Read the model definition and answer for the solid it produces. Units are mm, in the model's axes. A direction names the side the tool comes from. Coordinates: 2 decimals unless noted, no trailing zeros. Loops run counter-clockwise (first coordinate to the right, second up) from the corner with the lowest first, then second, coordinate; pieces in that order, holes last. Notation, with made-up numbers: M 41.5,4 L 96.5,4 A8 cw 96.5,14 Z; hole C -40,17.25 d4. An arc over 180 degrees is marked long. Put each result on its own line as item: value.
from build123d import *

# Parameters (mm, degrees)
SKETCH1_R               = 12.7
BOSS_EXTRUDE1_DEPTH     = 44.45
SKETCH5_R               = 12.7
SKETCH5_R_2             = 6.35
BOSS_EXTRUDE2_DEPTH     = 6.35
SKETCH8_W               = 6.35
SKETCH8_H               = 6.35
CUT_EXTRUDE1_DEPTH      = 51.8
CUT_EXTRUDE1_DEPTH_BACK = 51.8


with BuildPart() as part:
    # Sketch1 → Boss-Extrude1 (new body, symmetric)
    with BuildSketch(Plane.XY):
        with BuildLine():
            Line((-59.699595301, -246.884504011), (-38.184359795, -0.964236874))
            ThreePointArc((-38.184359795, -0.964236874), (-38.124009824, -0.108037848), (-38.092623076, 0.749711395))
            ThreePointArc((-38.092623076, 0.749711395), (0, 38.1), (38.092623076, 0.749711395))
            ThreePointArc((38.092623076, 0.749711395), (38.124009824, -0.108037848), (38.184359795, -0.964236874))
            Line((38.184359795, -0.964236874), (59.699595301, -246.884504011))
            ThreePointArc((59.699595301, -246.884504011), (0, -254), (-59.699595301, -246.884504011))
        make_face()
        Circle(SKETCH1_R, mode=Mode.SUBTRACT)
    extrude(amount=BOSS_EXTRUDE1_DEPTH, both=True)

    # Sketch5 → Boss-Extrude2 (add)
    with BuildSketch(Plane.XY.offset(44.45)):
        with BuildLine():
            Line((-223.779910529, -44.577802506), (-54.04268144, -3.827499177))
            ThreePointArc((-54.04268144, -3.827499177), (-42.924981025, 2.041131203), (-35.983316209, 12.522418081))
            ThreePointArc((-35.983316209, 12.522418081), (0, 38.1), (35.983316209, 12.522418081))
            ThreePointArc((35.983316209, 12.522418081), (42.924981025, 2.041131203), (54.04268144, -3.827499177))
            Line((54.04268144, -3.827499177), (223.779910529, -44.577802506))
            ThreePointArc((223.779910529, -44.577802506), (239.972758508, -56.795566669), (242.055998097, -76.973331649))
            ThreePointArc((242.055998097, -76.973331649), (0, -254), (-242.055998097, -76.973331649))
            ThreePointArc((-242.055998097, -76.973331649), (-239.972758508, -56.795566669), (-223.779910529, -44.577802506))
        make_face()
        Circle(SKETCH5_R, mode=Mode.SUBTRACT)
        with Locations((-117.332700629, -48.60079591)):
            Circle(SKETCH5_R_2, mode=Mode.SUBTRACT)
        with Locations((117.332700629, -48.60079591)):
            Circle(SKETCH5_R_2, mode=Mode.SUBTRACT)
    boss_extrude2 = extrude(amount=BOSS_EXTRUDE2_DEPTH)

    # Mirror1: Boss-Extrude2 across plane
    add(boss_extrude2.mirror(Plane.XY))

    # Sketch8 → Cut-Extrude1 (cut, two sides)
    with BuildSketch(Plane.XY) as cut_extrude1_sk:
        with Locations((0, 12.7)):
            Rectangle(SKETCH8_W, SKETCH8_H)
    extrude(amount=CUT_EXTRUDE1_DEPTH, mode=Mode.SUBTRACT)
    extrude(cut_extrude1_sk.sketch, amount=-CUT_EXTRUDE1_DEPTH_BACK, mode=Mode.SUBTRACT)


solid = part.part
1) Determine the mould class of faces 3 (the flat face through (3, -106, -50.8)), 4 (the cylindrical face through (120.75, -43.25, 47.58)), 5 (the flat face through (48.79, -122.2, 0.62)) for opening direction Z: released by +Z, released by -Z, zero draft, split by the parting line, or undercut.
Answer list:
face 3: released by -Z
face 4: zero draft
face 5: undercut
2) Find section D-D, the plane y = 21. Write down the section's boundary in (x, z), plus the area to 3 significant figures.
Answer list:
outline: M -31.79,-50.8 L 31.79,-50.8 L 31.79,50.8 L -31.79,50.8 Z
area: 6,460 mm^2
3) Find section B-B, the plane y = -227. Write down the section's boundary in (x, z), plus the area to 3 significant figures.
Answer list:
outline: M -113.96,-50.8 L 113.96,-50.8 L 113.96,-44.45 L 57.96,-44.45 L 57.96,44.45 L 113.96,44.45 L 113.96,50.8 L -113.96,50.8 L -113.96,44.45 L -57.96,44.45 L -57.96,-44.45 L -113.96,-44.45 Z
area: 13,200 mm^2
4) Find section C-C, the plane x = -47. Write down the section's boundary in (y, z).
Answer list:
outline: M -249.61,-50.8 L -0.97,-50.8 L -0.97,-44.45 L -101.73,-44.45 L -101.73,44.45 L -0.97,44.45 L -0.97,50.8 L -249.61,50.8 Z
5) Straight lines are drawn through the part: line 1 (Z direction, x = 121, y = -147); line 2 (X direction, y = 0, z = 5); line 3 (Y direction, x = -1.5, z = -26.5) (3 decimals). For each, find the intervals that lie inside material, in ascending order. Write a range as [from, to].
Answer list:
line 1: z = [-50.8, -44.45], [44.45, 50.8]
line 2: x = [-38.12, -12.7], [12.7, 38.12]
line 3: y = [-253.996, -12.611], [15.875, 38.07]
6) Which of the six approach directions +Z, -Z, +X, -X, +Y, -Y give full straight-line access (tool end or side, diameter ignored) to faces 1 (the flat face through (-49.093, -125.646, 0.622)), 2 (the cylindrical face through (-118.159, -42.305, -47.581))?
Answer list:
face 1: -X, +Y
face 2: +Z, -Z
7) Given pin 1 Ø14.5 at (x, y) = (117.33, -48.6) entering from -Z; pin 2 Ø6 at (y, z) = (-100.5, -4.5) entering from -X; pin 3 Ø2 at (y, z) = (-73.5, -38.5) entering from +X; pin 4 Ø1.8 at (y, z) = (13.5, -25.5) entering from +X, each flat-ended and moving along its own axis, determine where each tip first touches the part or whether it passes through.
Answer list:
pin 1: stops at z = -50.8
pin 2: stops at x = -47.16
pin 3: stops at x = 44.62
pin 4: stops at x = 35.96
8) Find section A-A, the plane z = 8. Write down the section's boundary in (x, y) (1 decimal), plus the area to 3 significant figures.
Answer list:
outline: M -59.7,-246.9 A254 ccw 59.7,-246.9 L 38.2,-1 A25.4 cw 38.1,0.7 A38.1 ccw -38.1,0.7 A25.4 cw -38.2,-1 Z; hole M -3.2,12.3 A12.7 ccw long 3.2,12.3 L 3.2,15.9 L -3.2,15.9 Z
area: 26,500 mm^2
